Input: part model. Units: mm. Frame: model coordinates. A direction names the side the tool comes from. Give positions to 0.01 mm unless a question says otherwise; leave off trailing zeros. Loops run counter-clockwise (first coordinate to the right, second up) from the corner with the lowest first, then second, coordinate; pieces in that order, holes last. Notation, with made-up numbers: (18, 52.5) -> (34, 52.5) arc R34 ccw to (34, 87.5) -> close; hole circle Ø2 at (-7.5, 59.5). An arc over 180 degrees is marked (long way). Answer as a JSON object with one key per item and string values.
```python
from build123d import *

# Parameters (mm, degrees)
F1_DEPTH = 10.16
F2_W     = 12.7
F2_H     = 25.4
F3_DEPTH = 15.24
F4_W     = 12.7
F4_H     = 12.7
F5_DEPTH = 9.525
F6_DEPTH = 3.81


with BuildPart() as f1:
    # F0 (on Top) → F1 (new body)
    with BuildSketch(Plane.XY):
        with BuildLine():
            Line((15.875, -19.05), (15.875, 19.05))
            Line((15.875, 19.05), (-15.875, 19.05))
            ThreePointArc((-15.875, 19.05), (-2.4046158184, 13.4703841816), (3.175, 0))
            ThreePointArc((3.175, 0), (-2.4046158184, -13.4703841816), (-15.875, -19.05))
            Line((-15.875, -19.05), (15.875, -19.05))
        make_face()
        with BuildLine():
            ThreePointArc((3.175, 0), (-2.4046158184, 13.4703841816), (-15.875, 19.05))
            Line((-15.875, 19.05), (-15.875, 9.525))
            ThreePointArc((-15.875, 9.525), (-9.1398079092, 6.7351920908), (-6.35, 0))
            ThreePointArc((-6.35, 0), (-9.1398079092, -6.7351920908), (-15.875, -9.525))
            Line((-15.875, -9.525), (-15.875, -19.05))
            ThreePointArc((-15.875, -19.05), (-2.4046158184, -13.4703841816), (3.175, 0))
        make_face()
        with BuildLine():
            Line((-15.875, 9.525), (-15.875, 19.05))
            ThreePointArc((-15.875, 19.05), (-34.925, 0), (-15.875, -19.05))
            Line((-15.875, -19.05), (-15.875, -9.525))
            ThreePointArc((-15.875, -9.525), (-25.4, 0), (-15.875, 9.525))
        make_face()
    extrude(amount=F1_DEPTH)

    # F2 (on face) → F3 (join)
    with BuildSketch(Plane.XY.offset(10.16)):
        with Locations((9.525, -6.35)):
            Rectangle(F2_W, F2_H)
    extrude(amount=F3_DEPTH)

    # F4 (on face) → F5 (join)
    with BuildSketch(Plane.XY.offset(10.16)):
        with Locations((9.525, 12.7)):
            Rectangle(F4_W, F4_H)
    extrude(amount=F5_DEPTH)

    # F6 (add): a face of the model
    f6_faces = [f1.faces().sort_by_distance(p)[0] for p in [
        (9.525, -6.35, 25.4),
    ]]
    extrude(f6_faces, amount=F6_DEPTH)


solid = f1.part
```
Q1. Section C-C, the plane z = 6.5. Return the cut outline in (x, y) (3 decimals), then the cut area to 3 significant figures.
Evaluation:
{"outline": "(-15.875, -19.05) -> (15.875, -19.05) -> (15.875, 19.05) -> (-15.875, 19.05) arc R19.05 ccw to start; hole circle Ø19.05 at (-15.875, 0)", "area": "1,490 mm2"}
Q2. Access query for faces 4 (the flat face through (-12, 9, 10.16)), 5 (the flat face through (9, 13, 19.685)), 6 (the cylindrical face through (-34.92, 0.42, 5.01)). Directions: +Z, -Z, +X, -X, +Y, -Y. A direction counts if a zero-diameter tool reaches every point of the face in a straight line with its end or side. Return the directions, or none.
Evaluation:
{"face 4": "+Z, -X, +Y, -Y", "face 5": "+Z, +X, -X, +Y", "face 6": "+Z, -Z, -X"}
Q3. Section D-D, the plane x = 4.5. Return the cut outline in (y, z) (3 decimals), then the cut area to 3 significant figures.
Evaluation:
{"outline": "(-19.05, 0) -> (19.05, 0) -> (19.05, 19.685) -> (6.35, 19.685) -> (6.35, 29.21) -> (-19.05, 29.21) -> close", "area": "992 mm2"}
Q4. Pin query (flat end, axial travel): pin 1 (4 mm diameter, centred on x = 8.5, y = 14.5, fed in from +Z) (3 decimals); pin 2 (8 mm diameter, centred on y = -4.5, z = 17.5, fed in from -X) (3 decimals); pin 3 (4 mm diameter, centred on x = -27.5, z = 11.5, fed in from -Y). Return the tip coordinate at first contact, or that it passes through.
Evaluation:
{"pin 1": "stops at z = 19.685", "pin 2": "stops at x = 3.175", "pin 3": "stops at y = -16.13"}
Q5. Draft query along Y for faces 1 (the flat face through (15.875, 0, 14)), 2 (the cylindrical face through (-25.39, -0.42, 5.01)), 3 (the flat face through (9, 6.35, 24)). Return one class per face: +Y half, -Y half, draft (parallel to the pull), parting line (faces both ways), or undercut.
Evaluation:
{"face 1": "draft", "face 2": "undercut", "face 3": "+Y half"}
Q6. Section A-A, the plane y = 0. Return the cut outline in (x, z) (3 decimals), then the cut area to 3 significant figures.
Evaluation:
{"outline": "(-34.925, 0) -> (-25.4, 0) -> (-25.4, 10.16) -> (-34.925, 10.16) -> close; (-6.35, 0) -> (15.875, 0) -> (15.875, 29.21) -> (3.175, 29.21) -> (3.175, 10.16) -> (-6.35, 10.16) -> close", "area": "565 mm2"}
Q7. Section B-B, the plane x = -10. Return the cut outline in (y, z), then the cut area to 3 significant figures.
Evaluation:
{"outline": "(-19.05, 0) -> (-7.5, 0) -> (-7.5, 10.16) -> (-19.05, 10.16) -> close; (7.5, 0) -> (19.05, 0) -> (19.05, 10.16) -> (7.5, 10.16) -> close", "area": "235 mm2"}
Q8. Ray query, line 1 along Z through (x, y) = (-30.5, -7); line 2 along Z through (x, y) = (6, 10) (3 decimals); line 3 along X through (y, z) = (0.5, 3) (3 decimals). Return the intervals inside material, ascending.
Evaluation:
{"line 1": "z = 0 to 10.16", "line 2": "z = 0 to 19.685", "line 3": "x = -34.918 to -25.387, -6.363 to 15.875"}
